Check sheet for the drawn part. Datum: minimum x, y, z corner. Units: mm. A direction names the side the tool comes from. Give positions to 0.01 mm unless a question says otherwise; leave off trailing zeros. Order: outer loops, then holes, each group sorted by start corner. A loop starts at its lowest first (then second) coordinate and runs counter-clockwise, first axis right, second up.
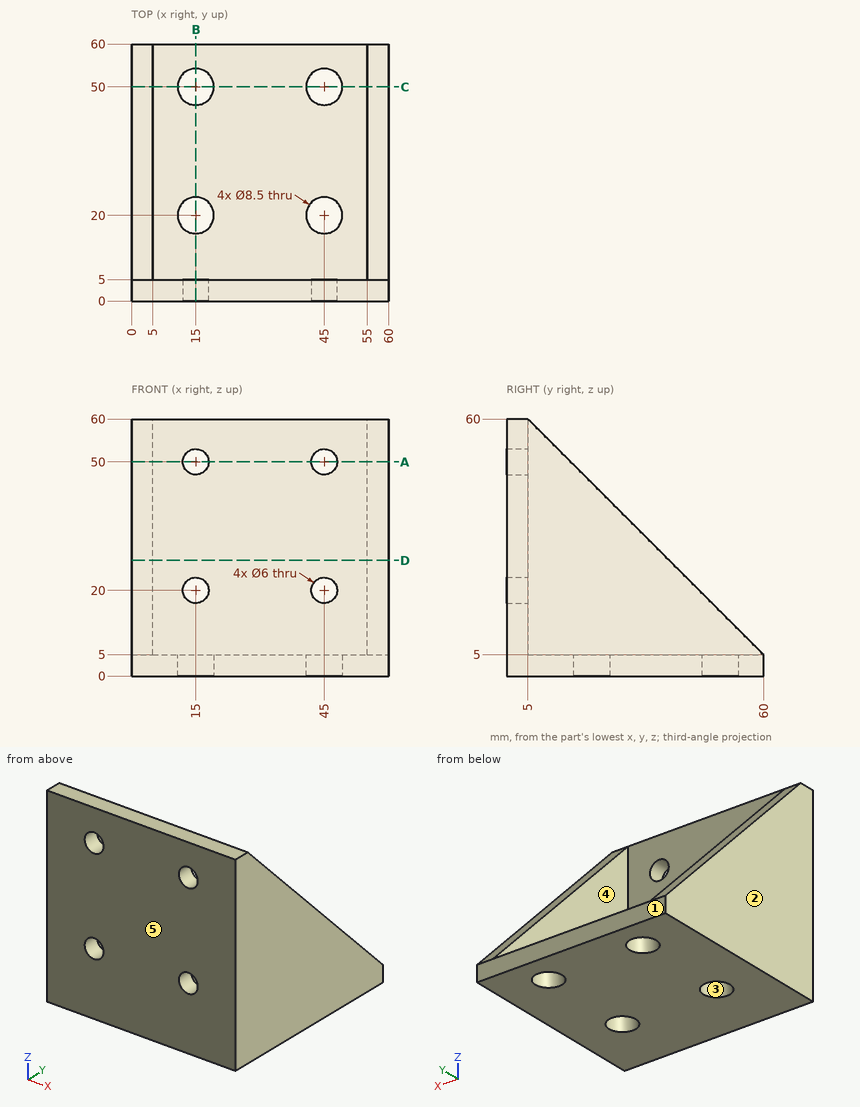
Q1. Material ranges on line 1 (Z direction, x = 15, y = 2); line 2 (Y direction, x = 45, z = 3.1); line 3 (X direction, y = 29.5, z = 7), recorded low to high.
Q2. Sectioned sample at B-B, the plane x = 15. Record the cut outline in (y, z), plus the area to 3 significant figures.
Q3. Go/stop test with flat-tipped pins: P1, Ø1, axis at x = 31, z = 42, coming from the +Y side; P2, Ø3.5, axis at x = 15, z = 50, coming from the -Y side; P3, Ø1.5, axis at x = 21.5, y = 25, coming from the +Z side. Record where each tip stops, or that it passes through.
Q4. Sectioned sample at D-D, the plane z = 27. Record the cut outline in (x, y), plus the area to 3 significant figures.
Q5. Sectioned sample at C-C, the plane y = 50. Record the cut outline in (x, z).
Q6. Tool access check on the marked faces 4 and 5. Record the directions out of +Z, -Z, +X, -X, +Y, -Y that give a thin tool (end or side, any length) a straight path to the whole face; none if there is none.
Q7. Draft check along X on the marked faces 1, 2 and 3. Enter one of: pulls with the +X half, pulls with the -X half, needs draft (parallel to the pull), parting line crosses it, or undercut.
Q8. Sectioned sample at A-A, the plane z = 50. Record the cut outline in (x, y).
Filled in:
1. line 1: z = 0 to 17, 23 to 47, 53 to 60
1. line 2: y = 0 to 15.75, 24.25 to 45.75, 54.25 to 60
1. line 3: x = 0 to 5, 55 to 60
2. outline: (0, 0) - (15.75, 0) - (15.75, 5) - (5, 5) - (5, 17) - (0, 17) - close; (0, 23) - (5, 23) - (5, 47) - (0, 47) - close; (0, 53) - (5, 53) - (5, 60) - (0, 60) - close; (24.25, 0) - (45.75, 0) - (45.75, 5) - (24.25, 5) - close; (54.25, 0) - (60, 0) - (60, 5) - (54.25, 5) - close
2. area: 430 mm2
3. P1: stops at y = 5
3. P2: passes through
3. P3: stops at z = 5
4. outline: (0, 0) - (60, 0) - (60, 38) - (55, 38) - (55, 5) - (5, 5) - (5, 38) - (0, 38) - close
4. area: 630 mm2
5. outline: (0, 0) - (10.75, 0) - (10.75, 5) - (5, 5) - (5, 15) - (0, 15) - close; (19.25, 0) - (40.75, 0) - (40.75, 5) - (19.25, 5) - close; (49.25, 0) - (60, 0) - (60, 15) - (55, 15) - (55, 5) - (49.25, 5) - close
6. face 4: +Z, +Y
6. face 5: +Z, -Z, +X, -X, -Y
7. face 1: needs draft
7. face 2: pulls with the -X half
7. face 3: undercut
8. outline: (0, 0) - (12, 0) - (12, 5) - (5, 5) - (5, 15) - (0, 15) - close; (18, 0) - (42, 0) - (42, 5) - (18, 5) - close; (48, 0) - (60, 0) - (60, 15) - (55, 15) - (55, 5) - (48, 5) - close
